Could you check a few things on this model? Use its own coordinates, in mm. A direction names the side the tool comes from. Round coordinates to 2 decimals unless told otherwise and drop trailing zeros. Loops run counter-clockwise (first coordinate to the right, second up) from the corner with the lowest first, then second, coordinate; pieces in that order, holes last. Notation, with made-up numbers: (22.5, -29) -> (57.5, -29) arc R22 cw to (57.5, -19) -> close; hole circle Ø8 at (61.25, 43.5). An arc over 180 degrees is marked (long way). Write each question's results on one line, items separated by ' | '.
from build123d import *

# Parameters (mm, degrees)
SKIZZE2_W                       = 8
SKIZZE2_H                       = 8
SKIZZE2_W_2                     = 7.4
SKIZZE2_H_2                     = 7.4
AUFSATZ_LINEAR_AUSTRAGEN1_DEPTH = 0.6
SKIZZE5_W                       = 8
SKIZZE5_H                       = 8
AUFSATZ_LINEAR_AUSTRAGEN3_DEPTH = 0.35
SKIZZE4_W                       = 8
SKIZZE4_H                       = 8
AUFSATZ_LINEAR_AUSTRAGEN2_DEPTH = 0.3
SKIZZE7_W                       = 8
SKIZZE7_H                       = 8
SKIZZE7_R                       = 2.8
AUFSATZ_LINEAR_AUSTRAGEN4_DEPTH = 1.8
SKIZZE8_R                       = 3.8
SKIZZE8_R_2                     = 2.8
AUFSATZ_LINEAR_AUSTRAGEN5_DEPTH = 0.9
FASE1_SIZE                      = 0.4


with BuildPart() as part:
    # Skizze2 → Aufsatz-Linear austragen1 (new body)
    with BuildSketch(Plane(origin=(0, 0, 0), x_dir=(1, 0, 0), z_dir=(0, 1, 0))):
        Rectangle(SKIZZE2_W, SKIZZE2_H)
        Rectangle(SKIZZE2_W_2, SKIZZE2_H_2, mode=Mode.SUBTRACT)
    extrude(amount=AUFSATZ_LINEAR_AUSTRAGEN1_DEPTH)

    # Skizze5 → Aufsatz-Linear austragen3 (add)
    with BuildSketch(Plane(origin=(0, 0.6, 0), x_dir=(1, 0, 0), z_dir=(0, 1, 0))):
        Rectangle(SKIZZE5_W, SKIZZE5_H)
        with BuildLine():
            Line((-2.764589803, 3.2), (2.764589803, 3.2))
            ThreePointArc((2.764589803, 3.2), (3.347487373, 3.347487373), (3.2, 2.764589803))
            Line((3.2, 2.764589803), (3.2, -2.764589803))
            ThreePointArc((3.2, -2.764589803), (3.347487373, -3.347487373), (2.764589803, -3.2))
            Line((2.764589803, -3.2), (-2.764589803, -3.2))
            ThreePointArc((-2.764589803, -3.2), (-3.347487373, -3.347487373), (-3.2, -2.764589803))
            Line((-3.2, -2.764589803), (-3.2, 2.764589803))
            ThreePointArc((-3.2, 2.764589803), (-3.347487373, 3.347487373), (-2.764589803, 3.2))
        make_face(mode=Mode.SUBTRACT)
    extrude(amount=AUFSATZ_LINEAR_AUSTRAGEN3_DEPTH)

    # Skizze4 → Aufsatz-Linear austragen2 (add)
    with BuildSketch(Plane(origin=(0, 0.95, 0), x_dir=(1, 0, 0), z_dir=(0, 1, 0))):
        Rectangle(SKIZZE4_W, SKIZZE4_H)
        with BuildLine():
            Line((-1.55, 2.15), (1.55, 2.15))
            ThreePointArc((1.55, 2.15), (1.974264069, 1.974264069), (2.15, 1.55))
            Line((2.15, 1.55), (2.15, -1.55))
            ThreePointArc((2.15, -1.55), (1.974264069, -1.974264069), (1.55, -2.15))
            Line((1.55, -2.15), (-1.55, -2.15))
            ThreePointArc((-1.55, -2.15), (-1.974264069, -1.974264069), (-2.15, -1.55))
            Line((-2.15, -1.55), (-2.15, 1.55))
            ThreePointArc((-2.15, 1.55), (-1.974264069, 1.974264069), (-1.55, 2.15))
        make_face(mode=Mode.SUBTRACT)
    extrude(amount=AUFSATZ_LINEAR_AUSTRAGEN2_DEPTH)

    # Skizze7 → Aufsatz-Linear austragen4 (add)
    with BuildSketch(Plane(origin=(0, 1.25, 0), x_dir=(1, 0, 0), z_dir=(0, 1, 0))):
        Rectangle(SKIZZE7_W, SKIZZE7_H)
        Circle(SKIZZE7_R, mode=Mode.SUBTRACT)
    extrude(amount=AUFSATZ_LINEAR_AUSTRAGEN4_DEPTH)

    # Skizze8 → Aufsatz-Linear austragen5 (add)
    with BuildSketch(Plane(origin=(0, 3.05, 0), x_dir=(1, 0, 0), z_dir=(0, 1, 0))):
        Circle(SKIZZE8_R)
        Circle(SKIZZE8_R_2, mode=Mode.SUBTRACT)
    extrude(amount=AUFSATZ_LINEAR_AUSTRAGEN5_DEPTH)

    # Fase1
    fase1_edges = [part.edges().sort_by_distance(p)[0] for p in [
        (-2.8, 3.95, 0),
    ]]
    chamfer(fase1_edges, length=FASE1_SIZE)


solid = part.part
1) If we mould it in two halves opening along X, with no side actions, what happens to faces 1 (the cylindrical face through (-3.796, 3.494, -0.167)), 2 (the flat face through (-4, 2, 0)), 3 (the cylindrical face through (-2.8, 2.4, -0.1))? For each: released by +X, released by -X, zero draft, split by the parting line, or undercut.
Model answer:
face 1: split by the parting line | face 2: released by -X | face 3: undercut
2) I want a section at D-D, the plane y = 3.75. Write out the boundary of the cut face in (x, z).
Model answer:
outline: circle Ø7.6 at (0, 0); hole circle Ø6 at (0, 0)
3) I need wall thicknesses on line 1 (X direction, y = 0.8, z = -3.1); line 2 (Z direction, x = 0, y = 3.15); line 3 (X direction, y = 0.2, z = 1). Which ranges of each line are inside material? Lowest first, please.
Model answer:
line 1: x = -4 to -3.45, 3.45 to 4 | line 2: z = -3.8 to -2.8, 2.8 to 3.8 | line 3: x = -4 to -3.7, 3.7 to 4
4) I'm going to push flat-ended pins straight in: pin 1 (1 mm diameter, centred on x = 1, z = -2, fed in from +Y); pin 2 (1 mm diameter, centred on x = -1.5, z = -1.5, fed in from +Y). Where does each tip first touch, or does it pass through?
Model answer:
pin 1: stops at y = 1.25 | pin 2: passes through
5) For faces 4 (the flat face through (-0.05, 0.95, -2.35)), 5 (the flat face through (-2, 3.95, 3)), which set-ups out of +Z, -Z, +X, -X, +Y, -Y let a thin tool reach every point of the face, with its end or its side?
Model answer:
face 4: -Y | face 5: +Z, -Z, +X, -X, +Y
6) I want a section at A-A, the plane z = 0. Write out the boundary of the cut face in (x, y).
Model answer:
outline: (-4, 0) -> (-3.7, 0) -> (-3.7, 0.6) -> (-3.2, 0.6) -> (-3.2, 0.95) -> (-2.15, 0.95) -> (-2.15, 1.25) -> (-2.8, 1.25) -> (-2.8, 3.55) -> (-3.2, 3.95) -> (-3.8, 3.95) -> (-3.8, 3.05) -> (-4, 3.05) -> close; (2.15, 0.95) -> (3.2, 0.95) -> (3.2, 0.6) -> (3.7, 0.6) -> (3.7, 0) -> (4, 0) -> (4, 3.05) -> (3.8, 3.05) -> (3.8, 3.95) -> (3.2, 3.95) -> (2.8, 3.55) -> (2.8, 1.25) -> (2.15, 1.25) -> close
7) I want a section at B-B, the plane x = 0. Write out the boundary of the cut face in (y, z).
Model answer:
outline: (0, -4) -> (3.05, -4) -> (3.05, -3.8) -> (3.95, -3.8) -> (3.95, -3.2) -> (3.55, -2.8) -> (1.25, -2.8) -> (1.25, -2.15) -> (0.95, -2.15) -> (0.95, -3.2) -> (0.6, -3.2) -> (0.6, -3.7) -> (0, -3.7) -> close; (0, 3.7) -> (0.6, 3.7) -> (0.6, 3.2) -> (0.95, 3.2) -> (0.95, 2.15) -> (1.25, 2.15) -> (1.25, 2.8) -> (3.55, 2.8) -> (3.95, 3.2) -> (3.95, 3.8) -> (3.05, 3.8) -> (3.05, 4) -> (0, 4) -> close
8) I want a section at C-C, the plane y = 1.9. Write out the boundary of the cut face in (x, z).
Model answer:
outline: (-4, -4) -> (4, -4) -> (4, 4) -> (-4, 4) -> close; hole circle Ø5.6 at (0, 0)
